from build123d import *

# Parameters (mm, degrees)
F0_R      = 36.5125
F1_DEPTH  = 31.75
F2_D      = 57.785
F3_D      = 58.674
F3_DEPTH  = 9.779
F3_TIP    = 17.6274479804
F4_SIZE   = 0.635
F7_W      = 19.3039988202
F7_H      = 4.572
F8_ANGLE  = 90
F9_W      = 30.988
F9_H      = 9.652
F10_DEPTH = 50.8


with BuildPart() as f1:
    # F0 (on Top) → F1 (new body)
    with BuildSketch(Plane.XY):
        Circle(F0_R)
    extrude(amount=-F1_DEPTH)

    # F2 (through all)
    with Locations(Plane.XY):
        with Locations((0, 0)):
            Hole(F2_D / 2)

    # F3
    with Locations(Plane.XY):
        with Locations((0, 0)):
            Hole(F3_D / 2, depth=F3_DEPTH)
            with Locations((0, 0, -(F3_DEPTH + F3_TIP / 2))):  # 118° drill point
                Cone(0, F3_D / 2, F3_TIP, mode=Mode.SUBTRACT)

    # F4
    f4_edges = [f1.edges().sort_by_distance(p)[0] for p in [
        (-36.5125, 0, 0),
    ]]
    chamfer(f4_edges, length=F4_SIZE)

    # F7 (on Front) → F8 (revolve, cut)
    with BuildSketch(Plane.XZ):
        with Locations((-33.327289857, -7.366)):
            Rectangle(F7_W, F7_H)
        with Locations((33.327289857, -7.366)):
            Rectangle(F7_W, F7_H)
    revolve(axis=Axis((0, 0, -17.7771920571), (0, 0, 1)), revolution_arc=F8_ANGLE, mode=Mode.SUBTRACT)

    # F9 (on Front) → F10 (cut, symmetric)
    with BuildSketch(Plane.XZ):
        with Locations((0, -4.826)):
            Rectangle(F9_W, F9_H)
    extrude(amount=F10_DEPTH, both=True, mode=Mode.SUBTRACT)


solid = f1.part
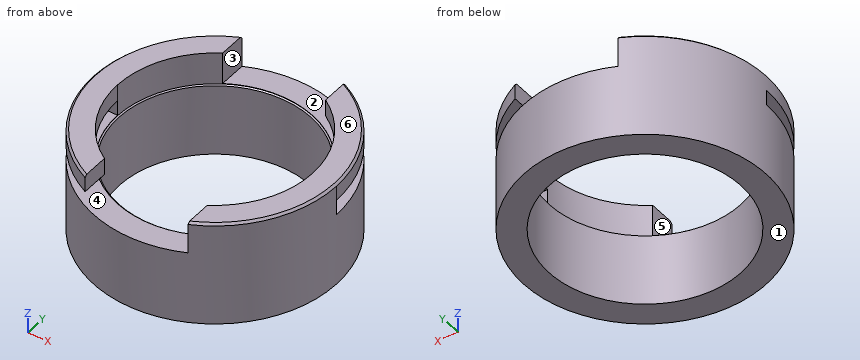
The listing builds one solid part. Answer for the finished solid, in the listing's coordinates (mm). Face numbers are marked on the shaded views. A direction names the side the tool comes from. Coordinates: 2 decimals unless noted, no trailing zeros. Write each loop counter-clockwise with the first axis right and the second up, starting at its lowest first coordinate (ties: lowest second). Pieces come first, ordered by that corner, then holes. Notation, with made-up numbers: (56.25, 49.5) - (99.25, 49.5) arc R14 cw to (99.25, 72.5) - close; hole circle Ø9 at (36, 7). An arc over 180 degrees is marked (long way). Return JSON: item names as keys, results as strings.
1. Which of the six approach directions +Z, -Z, +X, -X, +Y, -Y give full straight-line access (tool end or side, diameter ignored) to the marked faces 5 and 6?
Final values:
{"face 5": "+Z, +Y, -Y", "face 6": "+Z, +X, -X, +Y, -Y"}
2. For a pull along Z with two mould halves and no side action, classify the marked faces 1, 2, 3 and 4 as +Z half, -Z half, draft (parallel to the pull), parting line (faces both ways), or undercut.
Final values:
{"face 1": "-Z half", "face 2": "undercut", "face 3": "draft", "face 4": "undercut"}
3. Each of these flat-tipped pins is pushed along its axis until it touches: pin 1 Ø5 at (x, z) = (-32.5, -6.5) entering from -Y; pin 2 Ø4 at (y, z) = (29, -3) entering from -X; pin 3 Ø6.5 at (y, z) = (29, -7) entering from +X. Where does it stop, or does it pass through?
Final values:
{"pin 1": "y = -20.16", "pin 2": "x = -24.58", "pin 3": "x = 25.25"}
4. The part is cut by section B-B on z = -23.5. Determine the outline of the cut face in (x, y) (1 decimal).
Final values:
{"outline": "circle Ø73 at (0, 0); hole circle Ø57.8 at (0, 0)"}
5. The part is cut by section A-A on x = 0. Determine the outline of the cut face in (y, z).
Final values:
{"outline": "(-36.51, -31.75) - (-28.89, -31.75) - (-28.89, -10.05) - (-29.34, -9.78) - (-29.34, -9.65) - (-36.51, -9.65) - close; (28.89, -31.75) - (36.51, -31.75) - (36.51, -9.65) - (29.34, -9.65) - (29.34, -9.78) - (28.89, -10.05) - close"}
6. Consider line 1 along X through (y, z) = (0, -3); line 2 along X through (y, z) = (0, -21.5). Determine where each line is inside the solid, lowest interval first.
Final values:
{"line 1": "-36.51 to -29.34, 29.34 to 36.51", "line 2": "-36.51 to -28.89, 28.89 to 36.51"}
7. The part is cut by section C-C on x = -27.5. Count the separate pieces of the cut face and the enclosed holes in it, then the cut area to 3 significant figures.
Final values:
{"separate pieces": "3", "enclosed holes": "0", "area": "872 mm^2"}
